Autodesk Inventor part; units mm, degrees
ref_plane "YZ Plane" through (0, 0, 0) normal (1, 0, 0) x (0, 1, 0)
ref_plane "XZ Plane" through (0, 0, 0) normal (0, 1, 0) x (-1, 0, 0)
ref_plane "XY Plane" through (0, 0, 0) normal (0, 0, 1) x (1, 0, 0)
sketch "Sketch1" plane through (0, 0, 0) normal (0, 0, 1) x (1, 0, 0)
  arc A0 (11.4498, 7.2597) -> (11.1125, 26.7625) centre (-3.0917, 16.7625) ccw
  arc A1 (11.4498, 7.2597) -> (13.9324, 5.1544) centre (12.8228, 6.3624) ccw
  arc A2 (13.9324, 5.1544) -> (16.1125, 26.7625) centre (2.8844, 17.1831) ccw
  line L0 (11.1125, 26.7625) -> (16.1125, 26.7625)
  point P0 (0, 0)
extrude "Extrusion1" add sketch "Sketch1" along normal blind 1
sketch "Sketch2" plane through (0, 0, 1) normal (0, 0, 1) x (1, 0, 0)
  arc A0 (11.4498, 7.2597) -> (11.1125, 26.7625) centre (-3.0917, 16.7625) ccw
  arc A1 (11.4498, 7.2597) -> (13.9324, 5.1544) centre (12.8228, 6.3624) ccw
  arc A2 (13.9324, 5.1544) -> (16.1125, 26.7625) centre (2.8844, 17.1831) ccw
  line L0 (16.1125, 26.7625) -> (11.1125, 26.7625)
  circle A3 centre (12.8228, 6.3624) radius 0.75
  point P0 (0, 0)
  dimension "d5" = 1.5
extrude "Extrusion2" add sketch "Sketch2" against normal blind 3.5 contours A3
fillet "Fillet1" radius 0.4 1 edges at (11.1125, 26.7625, 0.5)
properties material "Liga de Nickel-Copper 400"
Model file for the job. Use its own axes, mm. Round coordinates to 2 decimals unless told otherwise and drop trailing zeros. Loops run counter-clockwise (first coordinate to the right, second up) from the corner with the lowest first, then second, coordinate; pieces in that order, holes last. Notation, with made-up numbers: M 70.5,15.5 L 95.5,15.5 A32 ccw 95.5,42.5 Z; hole C 45,0.5 d1. An arc over 180 degrees is marked long. Put each result on its own line as item: value. Start each with the question number.
Item 1: Mould opens along Y. For faces 1 (the face through (15, 16, 1)), 2 (the face through (12.074, 6.395, -1.232)), 3 (the face through (14, 26.762, 0.5)), 4 (the face through (14.28, 16.83, 0.49)) say: released by +Y, released by -Y, zero draft, split by the parting line, or undercut.
Item 2: Drop flat-ended pins along their axis: P1, Ø2, axis at y = 19.5, z = 0, coming from the -X side; P2, Ø1.5, axis at x = 13.5, z = -0.5, coming from the -Y side; P3, Ø4, axis at x = 16, y = 20.5, coming from the -Z side. Give the stop position or say it passes through.
Item 3: Cut at B-B (y = 11.25). List the corners of the cut face in (x, z).
Item 4: Cut at A-A (z = 0.3). List the corners of the cut face in (x, y).
Item 5: Drill centre lines: line 1 along Z through (x, y) = (18.5, 20); line 2 along Y through (x, z) = (13.5, -2.05); line 3 along X through (y, z) = (24.5, 0.85). Where is each one in solid material? Low to high.
Item 6: Cut at C-C (x = 17.25). List the corners of the cut face in (y, z), then the cut area to 3 significant figures.
Item 7: Cut at D-D (z = -1.95). List the corners of the cut face in (x, y), then the cut area to 3 significant figures.
Answer block:
1. face 1: zero draft
1. face 2: split by the parting line
1. face 3: released by +Y
1. face 4: undercut
2. P1: x = 13.87
2. P2: y = 4.73
2. P3: z = 0
3. outline: M 13.38,0 L 18.1,0 L 18.1,1 L 13.38,1 Z
4. outline: M 11.45,7.26 A1.64 ccw 13.93,5.15 A16.33 ccw 16.11,26.76 L 11.86,26.76 A0.4 ccw 11.53,26.15 A17.37 cw Z
5. line 1: 0 to 1
5. line 2: 6.04 to 6.68
5. line 3: 12.46 to 17.49
6. outline: M 9.41,0 L 24.95,0 L 24.95,1 L 9.41,1 Z
6. area: 15.5 mm2
7. outline: C 12.82,6.36 d1.5
7. area: 1.77 mm2
